from build123d import *

# Parameters (mm, degrees)
SCHIZZO1_R                    = 10
ESTRUSIONE_ESTRUSIONE1_DEPTH  = 25
ESTRUSIONE_ESTRUSIONE2_START  = -16
SCHIZZO2_R                    = 12
SCHIZZO2_R_2                  = 10
ESTRUSIONE_ESTRUSIONE2_DEPTH  = 15
ESTRUSIONE_ESTRUSIONE3_START  = -19
SCHIZZO3_R                    = 15
SCHIZZO3_R_2                  = 10
ESTRUSIONE_ESTRUSIONE3_DEPTH  = 5
TAGLIO_ESTRUSIONE1_REACH      = 43.787
TAGLIO_ESTRUSIONE1_END_RADIUS = 12
TAGLIO_ESTRUSIONE1_START      = 9
SMUSSO1_SIZE                  = 0.5
SCHIZZO7_W                    = 1.2
SCHIZZO7_H                    = 1
SCHIZZO7_W_2                  = 1.5


with BuildPart() as part:
    # Schizzo1 → Estrusione-Estrusione1 (new, symmetric)
    with BuildSketch(Plane(origin=(0, 0, 0), x_dir=(0, 0, -1), z_dir=(1, 0, 0))):
        Circle(SCHIZZO1_R)
    extrude(amount=ESTRUSIONE_ESTRUSIONE1_DEPTH, both=True)

    # Schizzo2 → Estrusione-Estrusione2 (add)
    with BuildSketch(Plane(origin=(25, 0, 0), x_dir=(0, 0, -1), z_dir=(1, 0, 0)).offset(ESTRUSIONE_ESTRUSIONE2_START)):
        Circle(SCHIZZO2_R)
        Circle(SCHIZZO2_R_2, mode=Mode.SUBTRACT)
    extrude(amount=-ESTRUSIONE_ESTRUSIONE2_DEPTH)

    # Schizzo3 → Estrusione-Estrusione3 (add)
    with BuildSketch(Plane.ZY.offset(25).offset(ESTRUSIONE_ESTRUSIONE3_START)):
        Circle(SCHIZZO3_R)
        with Locations(Location((0, 0, 0), (0, 0, 180))):
            Circle(SCHIZZO3_R_2, mode=Mode.SUBTRACT)
    extrude(amount=ESTRUSIONE_ESTRUSIONE3_DEPTH)

    # Taglio-Estrusione1: up to this cylinder (the profile starts inside it)
    taglio_estrusione1_end = Plane(origin=(1, 0, 0), z_dir=(1, 0, 0)) * Cylinder(TAGLIO_ESTRUSIONE1_END_RADIUS, 112.574, mode=Mode.PRIVATE)
    # Schizzo5 → Taglio-Estrusione1 (cut, up to the surface)
    with BuildSketch(Plane(origin=(0, 0, 0), x_dir=(1, 0, 0), z_dir=(0, 1, 0)).offset(TAGLIO_ESTRUSIONE1_START), mode=Mode.PRIVATE) as taglio_estrusione1_sk1:
        with BuildLine():
            Line((-1.5, 4), (3.5, 4))
            ThreePointArc((3.5, 4), (7.5, 0), (3.5, -4))
            Line((3.5, -4), (-1.5, -4))
            ThreePointArc((-1.5, -4), (-5.5, 0), (-1.5, 4))
        make_face()
    taglio_estrusione1_tool1 = extrude(taglio_estrusione1_sk1.sketch, amount=TAGLIO_ESTRUSIONE1_REACH, mode=Mode.PRIVATE) & taglio_estrusione1_end
    add(taglio_estrusione1_tool1.solids().sort_by_distance((1, 9, 0))[0], mode=Mode.SUBTRACT)

    # Smusso1
    smusso1_edges = [part.edges().sort_by_distance(p)[0] for p in [
        (-6, 0, -15),
        (-11, 0, -15),
        (-25, 0, 10),
        (25, 0, 10),
        (9, 0, 12),
    ]]
    chamfer(smusso1_edges, length=SMUSSO1_SIZE)

    # Schizzo7 → Taglia-Rivoluzione1 (revolve, cut)
    with BuildSketch(Plane.XY, mode=Mode.PRIVATE) as taglia_rivoluzione1_sk:
        with Locations((21.6, 9.5)):
            Rectangle(SCHIZZO7_W, SCHIZZO7_H)
        with Locations((-22.75, 9.5)):
            Rectangle(SCHIZZO7_W_2, SCHIZZO7_H)
    revolve(taglia_rivoluzione1_sk.sketch.rotate(Axis((-25, 0, 0), (1, 0, 0)), 180), axis=Axis((-25, 0, 0), (1, 0, 0)), mode=Mode.SUBTRACT)


solid = part.part
Input: part model. Units: mm. Frame: model coordinates. A direction names the side the tool comes from. Give positions to 0.01 mm unless a question says otherwise; leave off trailing zeros. Order: outer loops, then holes, each group sorted by start corner. A loop starts at its lowest first (then second) coordinate and runs counter-clockwise, first axis right, second up. Notation, with made-up numbers: M -9,59.5 L 28,59.5 A18 cw 28,89.5 Z; hole C 83.5,17 d9. An arc over 180 degrees is marked long. Answer as a JSON object with one key per item and string values.
1. First-contact query: P1, Ø12, axis at x = -10, z = 9.5, coming from the -Y side; P2, Ø5, axis at x = -18, y = -5.5, coming from the +Z side; P3, Ø2.5, axis at x = 0.5, y = 10, coming from the -Z side. Flat tips, straight axial feed; report the tip coordinate or a pass-through.
Result sheet:
{"P1": "y = -14.59", "P2": "z = 9.54", "P3": "z = -8.21"}
2. Pull-direction query (X, two-part tool) for faces 1 (the flat face through (-23.5, -9, -2)), 2 (the flat face through (-25, 0, 0)), 3 (the cylindrical face through (-16.42, 3, -9.54)); classes: +X half, -X half, draft (parallel to the pull), parting line (faces both ways), or undercut.
Result sheet:
{"face 1": "undercut", "face 2": "-X half", "face 3": "draft"}
3. Cut plane A-A, the plane x = -13. Output: boundary loops of the cut face in (y, z).
Result sheet:
{"outline": "C 0,0 d20"}
4. Ray query, line 1 (X direction, y = 6.5, z = 6.5); line 2 (X direction, y = 10.25, z = -2.25); line 3 (X direction, y = -6, z = 12.25). Return the intervals inside material, ascending. Write a range as [from, to].
Result sheet:
{"line 1": "[-25, -23.5], [-22, 21], [22.2, 25]", "line 2": "[-11, -4.81], [6.81, 9]", "line 3": "[-11, -6]"}
5. Reachability of faces 4 (the cylindrical face through (-22.74, 6.633, -6.083)), 5 (the flat face through (-11, 10, 3)), 6 (the flat face through (-6, 12, 2)) from +Z, -Z, +X, -X, +Y, -Y: full face, straight path, thin tool, end or side. Return the list, or none.
Result sheet:
{"face 4": "none", "face 5": "-X", "face 6": "+X"}
